from build123d import *

# Parameters (mm, degrees)
F2_W      = 17
F2_H      = 20
F3_DEPTH  = 3
F5_DEPTH  = 17
F7_DEPTH  = 25
F8_W      = 6.6
F8_H      = 4
F9_DEPTH  = 25
F10_W     = 6.6
F10_H     = 4
F11_DEPTH = 25


with BuildPart() as f3:
    # F2 (on Top) → F3 (new body)
    with BuildSketch(Plane.XY):
        Rectangle(F2_W, F2_H)
    extrude(amount=F3_DEPTH)

    # F4 (on face) → F5 (join)
    with BuildSketch(Plane.XY.offset(3)):
        Polygon((-5.5, 7), (5.5, 7), (5.5, -10), (8.5, -10), (8.5, 10), (-8.5, 10), (-8.5, -10), (-5.5, -10), align=None)
    extrude(amount=F5_DEPTH)

    # F6 (on face) → F7 (intersect)
    with BuildSketch(Plane.YZ.offset(8.5)):
        Polygon((-10, 6), (-10, 0), (10, 0), (10, 20), (4, 20), (4, 19.5), (-9.5, 6), align=None)
    extrude(amount=-F7_DEPTH, mode=Mode.INTERSECT)

    # F8 (on face) → F9 (cut)
    with BuildSketch(Plane.XY.offset(3)):
        with BuildLine():
            ThreePointArc((3.3, 0.5), (0, 3.8), (-3.3, 0.5))
            Line((-3.3, 0.5), (3.3, 0.5))
        make_face()
        with Locations((0, -1.5)):
            Rectangle(F8_W, F8_H)
        with BuildLine():
            Line((3.3, -3.5), (-3.3, -3.5))
            ThreePointArc((-3.3, -3.5), (0, -6.8), (3.3, -3.5))
        make_face()
    extrude(amount=-F9_DEPTH, mode=Mode.SUBTRACT)

    # F10 (on face) → F11 (cut)
    with BuildSketch(Plane.XZ.offset(-7)):
        with BuildLine():
            ThreePointArc((-3.3, 9.5), (0, 6.2), (3.3, 9.5))
            Line((3.3, 9.5), (-3.3, 9.5))
        make_face()
        with Locations((0, 11.5)):
            Rectangle(F10_W, F10_H)
        with BuildLine():
            Line((-3.3, 13.5), (3.3, 13.5))
            ThreePointArc((3.3, 13.5), (0, 16.8), (-3.3, 13.5))
        make_face()
    extrude(amount=-F11_DEPTH, mode=Mode.SUBTRACT)


solid = f3.part
Build history of the part. All positions in model axes, mm. A direction names the side the tool comes from. Coordinates: 2 decimals unless noted, no trailing zeros. Order: outer loops, then holes, each group sorted by start corner. A loop starts at its lowest first (then second) coordinate and runs counter-clockwise, first axis right, second up. Notation, with made-up numbers: (-13, 89.5) - (28, 89.5) arc R24 cw to (28, 109.5) - close; hole circle Ø6 at (41, 24.25). An arc over 180 degrees is marked (long way). Write each question's results on one line, items separated by ' | '. Start each with the question number.
Item 1: Band-saw the part on A-A on z = 11. Write the cut outline in (x, y), and give its area (3 significant figures).
Item 2: Tool access for faces 1 (the face through (-0.1, 8.5, 6.2)), 2 (the face through (-0.1, -6.8, 1.5)), 3 (the face through (-4, -1, 3)): list every direction of +Z, -Z, +X, -X, +Y, -Y with a clear straight run to the whole face (end or side of a thin tool).
Item 3: Mould opens along Y. For faces 4 (the face through (-7, -2.7, 12.8)), 5 (the face through (4, 0, 0)), 6 (the face through (3.3, -2, 2)), 7 (the face through (-4, 10, 10)) say: released by +Y, released by -Y, zero draft, split by the parting line, or undercut.
Item 4: Band-saw the part on C-C on y = 5. Write the cut outline in (x, z).
Item 5: Band-saw the part on D-D on y = -5. Write the cut outline in (x, z).
Item 6: Band-saw the part on B-B on x = 0. Write the cut outline in (y, z).
Item 7: Wall check: probe 1 along X at (y, z) = (-1, 8.25); probe 2 along X at (y, z) = (-2.5, 2.75); probe 3 along Z at (x, y) = (3.5, 5.75). Give the ranges that are in metal, low to high. Write a range as [from, to].
Item 8: Flat gauge pins, fed straight in: pin 1 (8 mm diameter, centred on x = -0.5, y = -4, fed in from +Z); pin 2 (8.5 mm diameter, centred on y = -0.5, z = 15.5, fed in from -X); pin 3 (3 mm diameter, centred on y = -6, z = 12.5, fed in from -X). Where does each tip first touch, or does it go through?
Numbers:
1) outline: (-8.5, -4.5) - (-5.5, -4.5) - (-5.5, 7) - (-3.3, 7) - (-3.3, 10) - (-8.5, 10) - close; (3.3, 7) - (5.5, 7) - (5.5, -4.5) - (8.5, -4.5) - (8.5, 10) - (3.3, 10) - close | area: 100 mm^2
2) face 1: +Y, -Y | face 2: +Z, -Z | face 3: +Z, -Y
3) face 4: released by -Y | face 5: zero draft | face 6: undercut | face 7: released by +Y
4) outline: (-8.5, 0) - (8.5, 0) - (8.5, 20) - (5.5, 20) - (5.5, 3) - (-5.5, 3) - (-5.5, 20) - (-8.5, 20) - close
5) outline: (-8.5, 0) - (-2.94, 0) - (-2.94, 3) - (-5.5, 3) - (-5.5, 10.5) - (-8.5, 10.5) - close; (2.94, 0) - (8.5, 0) - (8.5, 10.5) - (5.5, 10.5) - (5.5, 3) - (2.94, 3) - close
6) outline: (-10, 0) - (-6.8, 0) - (-6.8, 3) - (-10, 3) - close; (3.8, 0) - (10, 0) - (10, 6.2) - (7, 6.2) - (7, 3) - (3.8, 3) - close; (7, 16.8) - (10, 16.8) - (10, 20) - (7, 20) - close
7) probe 1: [-8.5, -5.5], [5.5, 8.5] | probe 2: [-8.5, -3.3], [3.3, 8.5] | probe 3: [0, 3]
8) pin 1: z = 3 | pin 2: x = -8.5 | pin 3: through
